```python
from build123d import *

# Parameters (mm, degrees)
EXTRUDE_1_DEPTH     = 60
CUT_EXTRUDE_1_DEPTH = 55
SKETCH_3_R          = 20.789145554
SKETCH_3_R_2        = 17.789145554
EXTRUDE_2_DEPTH     = 10
SKETCH_4_R          = 9.072208596
CUT_EXTRUDE_5_DEPTH = 135.907375632


with BuildPart() as part:
    # 草图1 → 凸台-拉伸1 (new body)
    with BuildSketch(Plane.XY):
        with BuildLine():
            Line((0, 50), (60, 50))
            ThreePointArc((60, 50), (110, 0), (60, -50))
            Line((60, -50), (0, -50))
            ThreePointArc((0, -50), (-50, 0), (0, 50))
        make_face()
    extrude(amount=EXTRUDE_1_DEPTH)

    # 草图2 → 切除-拉伸1 (cut)
    with BuildSketch(Plane(origin=(0, 0, 0), x_dir=(-1, 0, 0), z_dir=(0, 0, -1))):
        with BuildLine():
            Line((-60, -47), (0, -47))
            ThreePointArc((0, -47), (47, 0), (0, 47))
            Line((0, 47), (-60, 47))
            ThreePointArc((-60, 47), (-107, 0), (-60, -47))
        make_face()
    extrude(amount=-CUT_EXTRUDE_1_DEPTH, mode=Mode.SUBTRACT)

    # 草图3 → 凸台-拉伸2 (add)
    with BuildSketch(Plane.XY.offset(60)):
        Circle(SKETCH_3_R)
        Circle(SKETCH_3_R_2, mode=Mode.SUBTRACT)
    extrude(amount=EXTRUDE_2_DEPTH)

    # 草图4 → 切除-拉伸5 (cut, through all)
    with BuildSketch(Plane.XY.offset(60)):
        Circle(SKETCH_4_R)
    extrude(amount=-CUT_EXTRUDE_5_DEPTH, mode=Mode.SUBTRACT)


solid = part.part
```
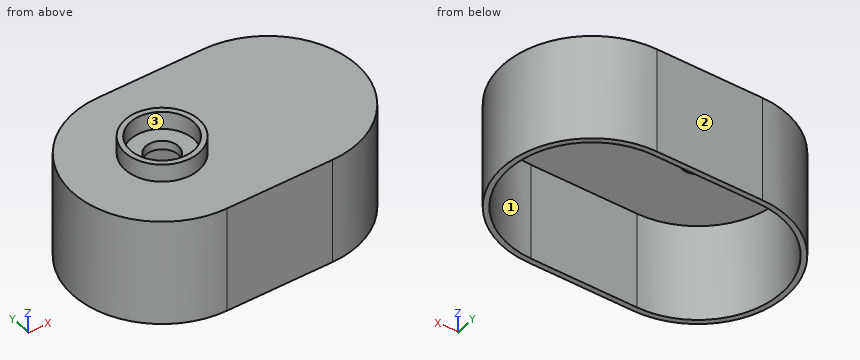
Here's how the part is built. I have some questions about the finished solid (model axes, mm). Face numbers are marked on the shaded views. A direction names the side the tool comes from. Coordinates: 2 decimals unless noted, no trailing zeros. Write each loop counter-clockwise with the first axis right and the second up, starting at its lowest first coordinate (ties: lowest second). Pieces come first, ordered by that corner, then holes. Notation, with made-up numbers: (78, -22.75) -> (101, -22.75) arc R17 ccw to (101, -13.75) -> close; hole circle Ø7 at (36, -15.75). An arc over 180 degrees is marked (long way). Use a Markdown table: item, result. Add a question column.
(1) I'm going to push flat-ended pins straight in: P1, Ø21, axis at x = 0, y = 0, coming from the +Z side; P2, Ø8, axis at y = 16, z = 15.5, coming from the +X side; P3, Ø10, axis at y = -17.5, z = 26.5, coming from the -X side. Where does each tip first touch, or does it pass through?
(2) If we section it at B-B, the plane z = 44: Write out the boundary of the cut face in (x, y).
(3) If we section it at C-C, the plane x = 5: Write out the boundary of the cut face in (y, z).
(4) If we section it at A-A, the plane y = 0: Write out the boundary of the cut face in (x, z).
(5) For the marked faces 1, 2 and 3, which set-ups out of +Z, -Z, +X, -X, +Y, -Y let a thin tool reach every point of the face, with its end or its side?
(6) If we section it at D-D, the plane x = 62: Write out the boundary of the cut face in (y, z), and give its area (3 significant figures).
(7) Please list where these lines run through material, in increasing order: line 1 (X direction, y = -1, z = 9.5); line 2 (Y direction, x = 0, z = 63); line 3 (Y direction, x = 39.5, z = 11.5).
Outcome:
| question | item | result |
|---|---|---|
| 1 | P1 | stops at z = 60 |
| 1 | P2 | stops at x = 108.54 |
| 1 | P3 | stops at x = -48.41 |
| 2 | outline | (0, -50) -> (60, -50) arc R50 ccw to (60, 50) -> (0, 50) arc R50 ccw to start; hole (0, -47) -> (60, -47) arc R47 ccw to (60, 47) -> (0, 47) arc R47 ccw to start |
| 3 | outline | (-50, 0) -> (-47, 0) -> (-47, 55) -> (-7.57, 55) -> (-7.57, 60) -> (-17.07, 60) -> (-17.07, 70) -> (-20.18, 70) -> (-20.18, 60) -> (-50, 60) -> close; (7.57, 55) -> (47, 55) -> (47, 0) -> (50, 0) -> (50, 60) -> (20.18, 60) -> (20.18, 70) -> (17.07, 70) -> (17.07, 60) -> (7.57, 60) -> close |
| 4 | outline | (-50, 0) -> (-47, 0) -> (-47, 55) -> (-9.07, 55) -> (-9.07, 60) -> (-17.79, 60) -> (-17.79, 70) -> (-20.79, 70) -> (-20.79, 60) -> (-50, 60) -> close; (9.07, 55) -> (107, 55) -> (107, 0) -> (110, 0) -> (110, 60) -> (20.79, 60) -> (20.79, 70) -> (17.79, 70) -> (17.79, 60) -> (9.07, 60) -> close |
| 5 | face 1 | -Z |
| 5 | face 2 | +Z, -Z, +X, -X, +Y |
| 5 | face 3 | +Z |
| 6 | outline | (-49.96, 0) -> (-46.96, 0) -> (-46.96, 55) -> (46.96, 55) -> (46.96, 0) -> (49.96, 0) -> (49.96, 60) -> (-49.96, 60) -> close |
| 6 | area | 830 mm^2 |
| 7 | line 1 | x = -49.99 to -46.99, 106.99 to 109.99 |
| 7 | line 2 | y = -20.79 to -17.79, 17.79 to 20.79 |
| 7 | line 3 | y = -50 to -47, 47 to 50 |
